from build123d import *

# Parameters (mm, degrees)
SKETCH1_W                = 400
SKETCH1_H                = 200
BOSS_EXTRUDE1_DEPTH      = 50
BOSS_EXTRUDE2_DEPTH      = 100
BOSS_EXTRUDE2_DEPTH_BACK = 100
CUT_EXTRUDE1_DEPTH       = 200
CUT_EXTRUDE1_DEPTH_BACK  = 200
SKETCH3_W                = 100
SKETCH3_H                = 185.844044806
CUT_EXTRUDE2_DEPTH       = 200
CUT_EXTRUDE2_DEPTH_BACK  = 200
SKETCH4_R                = 20


with BuildPart() as part:
    # Sketch1 → Boss-Extrude1 (new body)
    with BuildSketch(Plane(origin=(0, 0, 0), x_dir=(1, 0, 0), z_dir=(0, 1, 0))):
        Rectangle(SKETCH1_W, SKETCH1_H)
    extrude(amount=BOSS_EXTRUDE1_DEPTH)

    # Sketch2 → Boss-Extrude2 (add, two sides: drawn at the far end of the back side and taken through both)
    with BuildSketch(Plane.XY.offset(-BOSS_EXTRUDE2_DEPTH_BACK)):
        with BuildLine():
            Line((-100, 50), (100, 50))
            Line((100, 50), (200, 50))
            ThreePointArc((200, 50), (127.29182717, 109.861218113), (100, 200))
            Line((100, 200), (-100, 200))
            ThreePointArc((-100, 200), (-127.29182717, 109.861218113), (-200, 50))
            Line((-200, 50), (-100, 50))
        make_face()
    extrude(amount=BOSS_EXTRUDE2_DEPTH + BOSS_EXTRUDE2_DEPTH_BACK)

    # Sketch3 → Cut-Extrude1 (cut, two sides: drawn at the far end of the back side and taken through both)
    with BuildSketch(Plane(origin=(0, 0, 0), x_dir=(0, 0, -1), z_dir=(1, 0, 0)).offset(-CUT_EXTRUDE1_DEPTH_BACK)):
        with Locations((0, 142.922022403)):
            Rectangle(SKETCH3_W, SKETCH3_H)
    extrude(amount=CUT_EXTRUDE1_DEPTH + CUT_EXTRUDE1_DEPTH_BACK, mode=Mode.SUBTRACT)

    # Sketch4 → Cut-Extrude2 (cut, two sides: drawn at the far end of the back side and taken through both)
    with BuildSketch(Plane.XY.offset(-CUT_EXTRUDE2_DEPTH_BACK)):
        with Locations(Location((-60, 150, 0), (0, 0, 270))):
            Circle(SKETCH4_R)
        with Locations(Location((60, 150, 0), (0, 0, 270))):
            Circle(SKETCH4_R)
    extrude(amount=CUT_EXTRUDE2_DEPTH + CUT_EXTRUDE2_DEPTH_BACK, mode=Mode.SUBTRACT)


solid = part.part
Geometry check sheet. Reference: the model listing, model coordinates, mm. A direction names the side the tool comes from. Give positions to 0.01 mm unless a question says otherwise; leave off trailing zeros. Loops run counter-clockwise (first coordinate to the right, second up) from the corner with the lowest first, then second, coordinate; pieces in that order, holes last. Notation, with made-up numbers: (-13.75, -39) -> (5.25, -39) arc R32 cw to (5.25, 0) -> close; hole circle Ø3 at (-38, 31). An arc over 180 degrees is marked (long way). Answer in a Markdown table with one row per item. Add a question column.
1) Cross-section at C-C on z = 57.5. Record the boundary of the cut face in (x, y).
2) Cross-section at A-A on y = 182.5. Record the boundary of the cut face in (x, z), and give its area (3 significant figures).
3) Draft check along X on faces 3 (the face through (-126.554, 110.977, 74.65)), 4 (the face through (128.04, 108.75, 74.65)), 5 (the face through (-59.12, 169.98, 74.65)). Enter one of: pulls with the +X half, pulls with the -X half, needs draft (parallel to the pull), parting line crosses it, or undercut.
4) Material ranges on probe 1 along Y at (x, z) = (60, -81); probe 2 along Z at (x, y) = (49, 170); probe 3 along X at (y, z) = (150, 77), recorded low to high. Write a range as from..to.
5) Gauge pin test, flat ends, axial feed: P1, Ø12, axis at x = 138, z = -61.5, coming from the +Y side; P2, Ø4, axis at y = 139.5, z = -50, coming from the +X side. Record the tip position at first contact, or that the pin passes through.
6) Set-up check for faces 1 (the face through (1, 200, 75)), 2 (the face through (-3, 107, 50)): record each of +Z, -Z, +X, -X, +Y, -Y from which the full face is reachable in a straight line by a thin tool's end or side.
7) Cross-section at B-B on x = 60. Record the boundary of the cut face in (y, z).
8) Cross-section at D-D on x = -165. Record the boundary of the cut face in (y, z), and give its area (3 significant figures).
Outcome:
| question | item | result |
|---|---|---|
| 1 | outline | (-200, 0) -> (200, 0) -> (200, 50) arc R162.5 cw to (100, 200) -> (-100, 200) arc R162.5 cw to (-200, 50) -> close; hole circle Ø40 at (-60, 150); hole circle Ø40 at (60, 150) |
| 2 | outline | (-100.95, -100) -> (100.95, -100) -> (100.95, -50) -> (-100.95, -50) -> close; (-100.95, 50) -> (100.95, 50) -> (100.95, 100) -> (-100.95, 100) -> close |
| 2 | area | 20,200 mm^2 |
| 3 | face 3 | pulls with the -X half |
| 3 | face 4 | pulls with the +X half |
| 3 | face 5 | undercut |
| 4 | probe 1 | y = 0..130, 170..200 |
| 4 | probe 2 | z = -100..-50, 50..100 |
| 4 | probe 3 | x = -107.88..-80, -40..40, 80..107.88 |
| 5 | P1 | stops at y = 103.17 |
| 5 | P2 | stops at x = 112.5 |
| 6 | face 1 | +Z, -Z, +X, -X, +Y |
| 6 | face 2 | +X, -X, +Y |
| 7 | outline | (0, -100) -> (130, -100) -> (130, -50) -> (50, -50) -> (50, 50) -> (130, 50) -> (130, 100) -> (0, 100) -> close; (170, -100) -> (200, -100) -> (200, -50) -> (170, -50) -> close; (170, 50) -> (200, 50) -> (200, 100) -> (170, 100) -> close |
| 8 | outline | (0, -100) -> (70, -100) -> (70, -50) -> (50, -50) -> (50, 50) -> (70, 50) -> (70, 100) -> (0, 100) -> close |
| 8 | area | 12,000 mm^2 |
